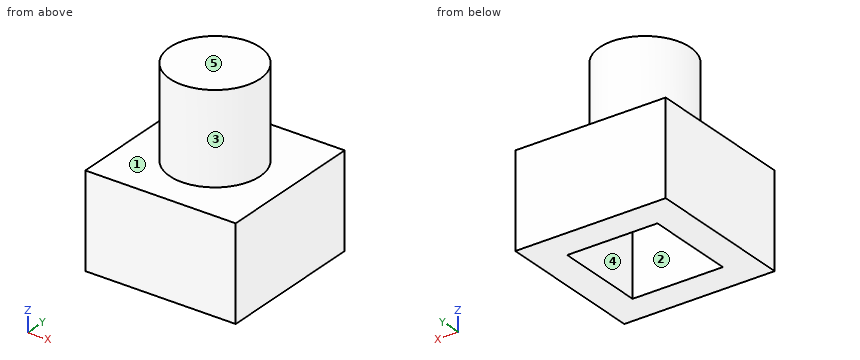
from build123d import *

# Parameters (mm, degrees)
F0_R     = 15
F1_DEPTH = 30
F2_W     = 50
F2_H     = 50
F3_DEPTH = 1
F4_W     = 50
F4_H     = 50
F4_W_2   = 30
F4_H_2   = 30
F5_DEPTH = 30


with BuildPart() as f1:
    # F0 (on Top) → F1 (new body)
    with BuildSketch(Plane.XY):
        Circle(F0_R)
    extrude(amount=F1_DEPTH)

    # F2 (on face) → F3 (join)
    with BuildSketch(Plane(origin=(0, 0, 0), x_dir=(1, 0, 0), z_dir=(0, 0, -1))):
        Rectangle(F2_W, F2_H)
        Polygon((15, 0), (15, -15), (0, -15), (-15, -15), (-15, 3.9e-09), (-15, 15), (0, 15), (15, 15), align=None, mode=Mode.SUBTRACT)
        with BuildLine():
            Line((0, -15), (15, -15))
            Line((15, -15), (15, 0))
            ThreePointArc((15, 0), (10.6066017178, -10.6066017178), (0, -15))
        make_face()
        with BuildLine():
            Line((-15, -15), (0, -15))
            ThreePointArc((0, -15), (-10.6066017192, -10.6066017164), (-15, 3.9e-09))
            Line((-15, 3.9e-09), (-15, -15))
        make_face()
        with BuildLine():
            ThreePointArc((-15, 3.9e-09), (-10.6066017192, -10.6066017164), (0, -15))
            ThreePointArc((0, -15), (10.6066017178, -10.6066017178), (15, 0))
            ThreePointArc((15, 0), (10.6066017178, 10.6066017178), (0, 15))
            ThreePointArc((0, 15), (-10.6066017164, 10.6066017192), (-15, 3.9e-09))
        make_face()
        with BuildLine():
            ThreePointArc((0, 15), (10.6066017178, 10.6066017178), (15, 0))
            Line((15, 0), (15, 15))
            Line((15, 15), (0, 15))
        make_face()
        with BuildLine():
            Line((-15, 15), (-15, 3.9e-09))
            ThreePointArc((-15, 3.9e-09), (-10.6066017164, 10.6066017192), (0, 15))
            Line((0, 15), (-15, 15))
        make_face()
    extrude(amount=F3_DEPTH)

    # F4 (on face) → F5 (join)
    with BuildSketch(Plane(origin=(0, 0, -1), x_dir=(1, 0, 0), z_dir=(0, 0, -1))):
        Rectangle(F4_W, F4_H)
        Rectangle(F4_W_2, F4_H_2, mode=Mode.SUBTRACT)
    extrude(amount=F5_DEPTH)


solid = f1.part
Geometry: final body of the model. Coordinates: model frame, mm. Face numbers are marked on the shaded views. A direction names the side the tool comes from. Coordinates: 2 decimals unless noted, no trailing zeros. Loops run counter-clockwise (first coordinate to the right, second up) from the corner with the lowest first, then second, coordinate; pieces in that order, holes last. Notation, with made-up numbers: M -36,78.25 L -1,78.25 A9 ccw -1,86.25 Z; hole C -17,-21.5 d3. An arc over 180 degrees is marked long. One line per item, written item: value. Start each with the question number.
1) Cut plane A-A (x = 0). Return loops of the section in (y, z).
2) Draft query along X for the marked faces 1, 2 and 3. Return one class per face: released by +X, released by -X, zero draft, split by the parting line, or undercut.
3) Reachability of the marked faces 4 and 5 from +Z, -Z, +X, -X, +Y, -Y: full face, straight path, thin tool, end or side. Return the list, or none.
4) Cut plane B-B (z = -22). Return loops of the section in (x, y).
5) Material intervals for L1, parallel to X at y = -12.5, z = -27; L2, parallel to Z at x = 17.5, y = 0, sorted ascending. Write a range as from..to.
6) Pin query (flat end, axial travel): P1, Ø2, axis at x = 13.5, y = -11.5, coming from the +Z side; P2, Ø1.5, axis at x = 14, y = 10.5, coming from the -Z side; P3, Ø1.5, axis at y = -1, z = 15.5, coming from the -X side. Return the tip coordinate at first contact, or that it passes through.
Evaluation:
1. outline: M -25,-31 L -15,-31 L -15,-1 L 15,-1 L 15,-31 L 25,-31 L 25,0 L 15,0 L 15,30 L -15,30 L -15,0 L -25,0 Z
2. face 1: zero draft
2. face 2: undercut
2. face 3: split by the parting line
3. face 4: -Z
3. face 5: +Z, +X, -X, +Y, -Y
4. outline: M -25,-25 L 25,-25 L 25,25 L -25,25 Z; hole M -15,-15 L 15,-15 L 15,15 L -15,15 Z
5. L1: -25..-15, 15..25
5. L2: -31..0
6. P1: z = 0
6. P2: z = -1
6. P3: x = -15
